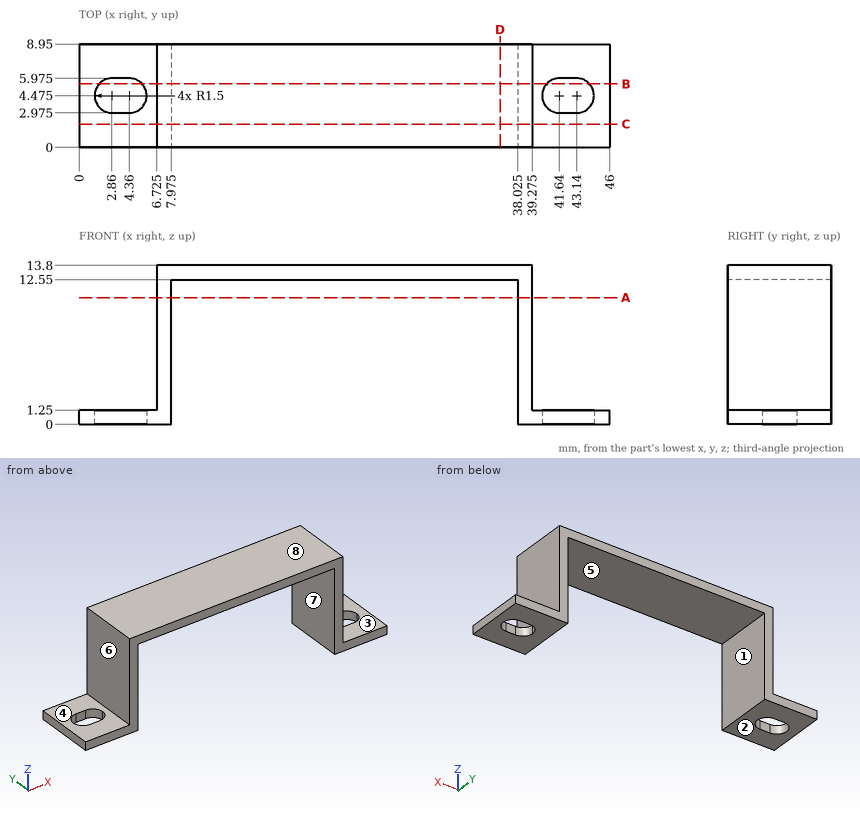
Can you work these out from the drawing? Everything is in mm from the part's minimum corner. A direction names the side the tool comes from. Coordinates: 2 decimals unless noted, no trailing zeros. Loops run counter-clockwise (first coordinate to the right, second up) from the corner with the lowest first, then second, coordinate; pieces in that order, holes last.
1) Which directions (+Z, -Z, +X, -X, +Y, -Y) give clear straight access to the entire face, cutting with the end or side of a thin tool? Please do the marked faces 1, 2, 3 and 4.
2) For pin 1 (1.5 mm diameter, centred on y = 8, z = 4.5, fed in from -X) (3 decimals); pin 2 (4.5 mm diameter, centred on y = 4, z = 9, fed in from +X) (3 decimals); pin 3 (2 mm diameter, centred on x = 4, y = 3.5, fed in from +Z), each with a flat end and sliding along its axis, tell me the tip position at first contact or that it passes through.
3) Imagine slicing it at C-C on y = 2. List the corners of the cut face in (x, z) for me (3 decimals), plus the area to 3 significant figures.
4) Imagine slicing it at A-A on z = 11. List the corners of the cut face in (x, y) for me (3 decimals).
5) Imagine slicing it at B-B on y = 5.5. List the corners of the cut face in (x, z) for me (3 decimals).
6) Imagine slicing it at D-D on x = 36.5. List the corners of the cut face in (y, z) for me.
7) Thinking about a two-plate mould opening in X: for the marked faces 5, 6, 7 and 8, which applies, pulls with the +X half, pulls with the -X half, needs draft (parallel to the pull), parting line crosses it, or undercut?
8) I need wall thicknesses on probe 1 along X at (y, z) = (2.75, 4) (3 decimals); probe 2 along Z at (x, y) = (33, 5.5); probe 3 along Y at (x, z) = (4, 0.5) (3 decimals). Which ranges of each line are inside material? Lowest first, please.
Completed:
1. face 1: -Z, +Y, -Y
1. face 2: -Z, +X, -X, +Y, -Y
1. face 3: +Z, +X, +Y, -Y
1. face 4: +Z, -X, +Y, -Y
2. pin 1: stops at x = 6.725
2. pin 2: stops at x = 39.275
2. pin 3: stops at z = 1.25
3. outline: (0, 0) - (7.975, 0) - (7.975, 12.55) - (38.025, 12.55) - (38.025, 0) - (46, 0) - (46, 1.25) - (39.275, 1.25) - (39.275, 13.8) - (6.725, 13.8) - (6.725, 1.25) - (0, 1.25) - close
3. area: 88.9 mm2
4. outline: (6.725, 0) - (7.975, 0) - (7.975, 8.95) - (6.725, 8.95) - close; (38.025, 0) - (39.275, 0) - (39.275, 8.95) - (38.025, 8.95) - close
5. outline: (0, 0) - (1.765, 0) - (1.765, 1.25) - (0, 1.25) - close; (5.455, 0) - (7.975, 0) - (7.975, 12.55) - (38.025, 12.55) - (38.025, 0) - (40.545, 0) - (40.545, 1.25) - (39.275, 1.25) - (39.275, 13.8) - (6.725, 13.8) - (6.725, 1.25) - (5.455, 1.25) - close; (44.235, 0) - (46, 0) - (46, 1.25) - (44.235, 1.25) - close
6. outline: (0, 12.55) - (8.95, 12.55) - (8.95, 13.8) - (0, 13.8) - close
7. face 5: undercut
7. face 6: pulls with the -X half
7. face 7: undercut
7. face 8: needs draft
8. probe 1: x = 6.725 to 7.975, 38.025 to 39.275
8. probe 2: z = 12.55 to 13.8
8. probe 3: y = 0 to 2.975, 5.975 to 8.95
